Part model, mm, in its own coordinate system. A direction names the side the tool comes from. Round coordinates to 2 decimals unless told otherwise and drop trailing zeros. Loops run counter-clockwise (first coordinate to the right, second up) from the corner with the lowest first, then second, coordinate; pieces in that order, holes last. Notation, with made-up numbers: M 36,40.5 L 80,40.5 A24 cw 80,57.5 Z; hole C -35.5,39.5 d1. An arc over 180 degrees is marked long. Put each result on its own line as item: value. Start each with the question number.
1) Slice it at D-D on z = -12.5. Give the cut face in (x, y), then the cut area to 3 significant figures.
2) Pull direction Z, two halves, no side cores. Call faces 1 (the flat face through (0, 2.54, -10)), 2 (the flat face through (-2.159, -15.5, -3.9)), 3 (the flat face through (13, -1, 0)): +Z half, -Z half, draft (parallel to the pull), parting line (faces both ways), or undercut.
3) Slice it at A-A on z = -5. Give the cut face in (x, y) (3 decimals).
4) Drop flat-ended pins along their axis: pin 1 Ø5 at (x, z) = (-17, -9.5) entering from -Y; pin 2 Ø1 at (y, z) = (-8, -1.5) entering from +X (3 decimals); pin 3 Ø1.4 at (x, y) = (-4, -12) entering from +Z. Give the stop position or say it passes through.
5) Which spindle directions (+Z, -Z, +X, -X, +Y, -Y) get a long thin tool onto all of the face, cutting with end or side? Do faces 4 (the flat face through (0, 0, -12)), 5 (the flat face through (-14, -1, 0)), 6 (the flat face through (3, -14.859, -3)), 7 (the flat face through (2.159, -15.5, -3.8)), 8 (the cylindrical face through (-0.07, -6.28, -8.89)). Say none if no direction does.
6) Probe line 1 along X through (y, z) = (0.5, -1.5) (3 decimals); line 2 along Y through (x, z) = (10, -15); line 3 along Y through (x, z) = (19, 0.25). List the from-to ranges inside material, lowest first.
7) Slice it at C-C on y = -11. Give the cut face in (x, z) (3 decimals).
8) Slice it at B-B on x = 0. Give the cut face in (y, z), then the cut area to 3 significant figures.
```python
from build123d import *

# Parameters (mm, degrees)
BOSS_EXTRUDE1_DEPTH = 2.54
BOSS_EXTRUDE2_START = -16.129
BOSS_EXTRUDE2_DEPTH = 18.669
SKETCH3_W           = 45.212
SKETCH3_H           = 3.81
BOSS_EXTRUDE3_DEPTH = 1.27
BOSS_EXTRUDE4_START = -16.129
BOSS_EXTRUDE4_DEPTH = 1.27


with BuildPart() as part:
    # Sketch1 → Boss-Extrude1 (new body)
    with BuildSketch(Plane(origin=(0, 0, 0), x_dir=(1, 0, 0), z_dir=(0, 1, 0))):
        with BuildLine():
            Line((22.606, 0), (22.606, 16.51))
            Line((22.606, 16.51), (-22.606, 16.51))
            Line((-22.606, 16.51), (-22.606, 0))
            Line((-22.606, 0), (-4.445, 0))
            Line((-4.445, 0), (-4.445, 5.715))
            ThreePointArc((-4.445, 5.715), (0, 10.16), (4.445, 5.715))
            Line((4.445, 5.715), (4.445, 0))
            Line((4.445, 0), (22.606, 0))
        make_face()
    extrude(amount=BOSS_EXTRUDE1_DEPTH)

    # Sketch2 → Boss-Extrude2 (add)
    with BuildSketch(Plane(origin=(0, 0, 0), x_dir=(1, 0, 0), z_dir=(0, 1, 0)).offset(BOSS_EXTRUDE2_START)):
        with BuildLine():
            Line((-4.445, 0), (-3.175, 0))
            Line((-3.175, 0), (-3.175, 5.715))
            ThreePointArc((-3.175, 5.715), (0, 8.89), (3.175, 5.715))
            Line((3.175, 5.715), (3.175, 0))
            Line((3.175, 0), (4.445, 0))
            Line((4.445, 0), (4.445, 5.715))
            ThreePointArc((4.445, 5.715), (0, 10.16), (-4.445, 5.715))
            Line((-4.445, 5.715), (-4.445, 0))
        make_face()
    extrude(amount=BOSS_EXTRUDE2_DEPTH)

    # Sketch3 → Boss-Extrude3 (add)
    with BuildSketch(Plane.XY):
        with Locations((0, 0.635)):
            Rectangle(SKETCH3_W, SKETCH3_H)
    extrude(amount=BOSS_EXTRUDE3_DEPTH)

    # Sketch4 → Boss-Extrude4 (add)
    with BuildSketch(Plane(origin=(0, 0, 0), x_dir=(1, 0, 0), z_dir=(0, 1, 0)).offset(BOSS_EXTRUDE4_START)):
        with BuildLine():
            Line((3.175, 5.715), (3.175, -1.27))
            Line((3.175, -1.27), (-3.175, -1.27))
            Line((-3.175, -1.27), (-3.175, 5.715))
            ThreePointArc((-3.175, 5.715), (0, 8.89), (3.175, 5.715))
        make_face()
        with BuildLine():
            Line((-2.159, 5.715), (-2.159, 1.982909029))
            ThreePointArc((-2.159, 1.982909029), (0, -0.176090971), (2.159, 1.982909029))
            Line((2.159, 1.982909029), (2.159, 5.715))
            ThreePointArc((2.159, 5.715), (0, 7.874), (-2.159, 5.715))
        make_face(mode=Mode.SUBTRACT)
    extrude(amount=BOSS_EXTRUDE4_DEPTH)


solid = part.part
```
Recorded:
1. outline: M -22.61,0 L 22.61,0 L 22.61,2.54 L -22.61,2.54 Z
1. area: 115 mm2
2. face 1: draft
2. face 2: undercut
2. face 3: -Z half
3. outline: M -22.606,0 L -4.445,0 L -4.445,-16.129 L -2.159,-16.129 L -2.159,-14.859 L -3.175,-14.859 L -3.175,2.54 L -22.606,2.54 Z; M 2.159,-16.129 L 4.445,-16.129 L 4.445,0 L 22.606,0 L 22.606,2.54 L 3.175,2.54 L 3.175,-14.859 L 2.159,-14.859 Z
4. pin 1: stops at y = 0
4. pin 2: stops at x = 4.445
4. pin 3: stops at z = 0
5. face 4: -Z, -Y
5. face 5: -Z, -X, -Y
5. face 6: +Z
5. face 7: +Y, -Y
5. face 8: +Y
6. line 1: x = -22.606 to -3.175, 3.175 to 22.606
6. line 2: y = 0 to 2.54
6. line 3: y = -1.27 to 2.54
7. outline: M -4.445,-5.715 A4.445 ccw 4.445,-5.715 L 4.445,0 L 3.175,0 L 3.175,-5.715 A3.175 cw -3.175,-5.715 L -3.175,0 L -4.445,0 Z
8. outline: M -16.13,-10.16 L 0,-10.16 L 0,-16.51 L 2.54,-16.51 L 2.54,-8.89 L -14.86,-8.89 L -14.86,-7.87 L -16.13,-7.87 Z; M -16.13,0.18 L -14.86,0.18 L -14.86,1.27 L -16.13,1.27 Z; M -1.27,0 L 2.54,0 L 2.54,1.27 L -1.27,1.27 Z
8. area: 47.4 mm2
